Part model, mm, in its own coordinate system. A direction names the side the tool comes from. Give positions to 0.01 mm unless a question says otherwise; leave off trailing zeros. Write each loop counter-clockwise with the first axis right and the second up, starting at its lowest first coordinate (ties: lowest second). Pieces come first, ordered by that corner, then holes. Notation, with made-up numbers: M 0.5,-32 L 54.5,-32 A26 ccw 54.5,6 Z; hole C 26,54 d10. An arc over 180 degrees is marked long. Answer as CSV lines item,"result". Start each with the question number.
1) Slice it at B-B, the plane y = -0.5. Give the cut face in (x, z).
2) Mould opens along X. For faces 1 (the flat face through (3.011, -0.525, 14.79)), 2 (the flat face through (0, 0, 0)), 3 (the flat face through (0, 4, -1)) say: pulls with the +X half, pulls with the -X half, needs draft (parallel to the pull), parting line crosses it, or undercut.
3) Pin check, flat tips, straight feed: pin 1 Ø1.5 at (x, y) = (0.5, 0) entering from -Z; pin 2 Ø0.7 at (x, z) = (2, 13.5) entering from -Y; pin 3 Ø1.2 at (x, z) = (2, 16.5) entering from +Y. Stop position of each tip, or through.
4) Wall check: line 1 along Y through (x, z) = (0, -1.3); line 2 along Z through (x, y) = (3.5, -1.5); line 3 along Y through (x, z) = (2, 10). Give the ranges that are in metal, low to high. Write a range as from..to.
5) Tool access for faces 4 (the flat face through (2, 2.5, 15)), 5 (the flat face through (2.5, -2, 15)), 6 (the flat face through (-2, 2.5, 15)), 7 (the cylindrical face through (-3.746, -0.165, -2.521)): list every direction of +Z, -Z, +X, -X, +Y, -Y with a clear straight run to the whole face (end or side of a thin tool).
6) Slice it at A-A, the plane z = 10. Give the cut face in (x, y), plus the area to 3 significant figures.
```python
from build123d import *

# Parameters (mm, degrees)
F1_DEPTH = 30
F2_R     = 4.25
F3_DEPTH = 5
F5_R     = 4.25
F5_R_2   = 3.75
F6_DEPTH = 3
F7_R     = 1.5
F8_DEPTH = 5


with BuildPart() as f1:
    # F0 (on Top) → F1 (new body)
    with BuildSketch(Plane.XY):
        Polygon((-2.5, -1.0355339059), (-2.5, -2.5), (-1.0355339059, -2.5), align=None)
        Polygon((-2.5, -1.0355339059), (-1.0355339059, -2.5), (1.0355339059, -2.5), (2.5, -1.0355339059), (2.5, 1.0355339059), (1.0355339059, 2.5), (-1.0355339059, 2.5), (-2.5, 1.0355339059), align=None)
        Polygon((1.0355339059, -2.5), (-1.0355339059, -2.5), (0, -3.5355339059), align=None)
        Polygon((-3.5355339059, 0), (-2.5, -1.0355339059), (-2.5, 1.0355339059), align=None)
        Polygon((2.5, -1.0355339059), (1.0355339059, -2.5), (2.5, -2.5), align=None)
        Polygon((-2.5, 2.5), (-2.5, 1.0355339059), (-1.0355339059, 2.5), align=None)
        Polygon((2.5, 1.0355339059), (2.5, -1.0355339059), (3.5355339059, 0), align=None)
        Polygon((0, 3.5355339059), (-1.0355339059, 2.5), (1.0355339059, 2.5), align=None)
        Polygon((1.0355339059, 2.5), (2.5, 1.0355339059), (2.5, 2.5), align=None)
    extrude(amount=F1_DEPTH)

    # F2 (on face) → F3 (join)
    with BuildSketch(Plane(origin=(0, 0, 0), x_dir=(1, 0, 0), z_dir=(0, 0, -1))):
        Circle(F2_R)
    extrude(amount=F3_DEPTH)

    # F5 (on offset) → F6 (cut)
    with BuildSketch(Plane(origin=(0, 0, -4), x_dir=(1, 0, 0), z_dir=(0, 0, -1))):
        Circle(F5_R)
        Circle(F5_R_2, mode=Mode.SUBTRACT)
    extrude(amount=-F6_DEPTH, mode=Mode.SUBTRACT)

    # F7 (on Top) → F8 (cut)
    with BuildSketch(Plane.XY):
        Circle(F7_R)
    extrude(amount=-F8_DEPTH, mode=Mode.SUBTRACT)


solid = f1.part
```
Found:
1,outline,"M -4.22,-5 L -1.41,-5 L -1.41,0 L 1.41,0 L 1.41,-5 L 4.22,-5 L 4.22,-4 L 3.72,-4 L 3.72,-1 L 4.22,-1 L 4.22,0 L 3.04,0 L 3.04,30 L -3.04,30 L -3.04,0 L -4.22,0 L -4.22,-1 L -3.72,-1 L -3.72,-4 L -4.22,-4 Z"
2,face 1,"pulls with the +X half"
2,face 2,"undercut"
2,face 3,"needs draft"
3,pin 1,"z = 0"
3,pin 2,"y = -2.5"
3,pin 3,"y = 2.5"
4,line 1,"-3.75..-1.5, 1.5..3.75"
4,line 2,"-5..-4, -1..0"
4,line 3,"-2.5..2.5"
5,face 4,"+Z, +X, +Y"
5,face 5,"+Z, +X, -Y"
5,face 6,"+Z, -X, +Y"
5,face 7,"none"
6,outline,"M -3.54,0 L -2.5,-1.04 L -2.5,-2.5 L -1.04,-2.5 L 0,-3.54 L 1.04,-2.5 L 2.5,-2.5 L 2.5,-1.04 L 3.54,0 L 2.5,1.04 L 2.5,2.5 L 1.04,2.5 L 0,3.54 L -1.04,2.5 L -2.5,2.5 L -2.5,1.04 Z"
6,area,"29.3 mm²"
